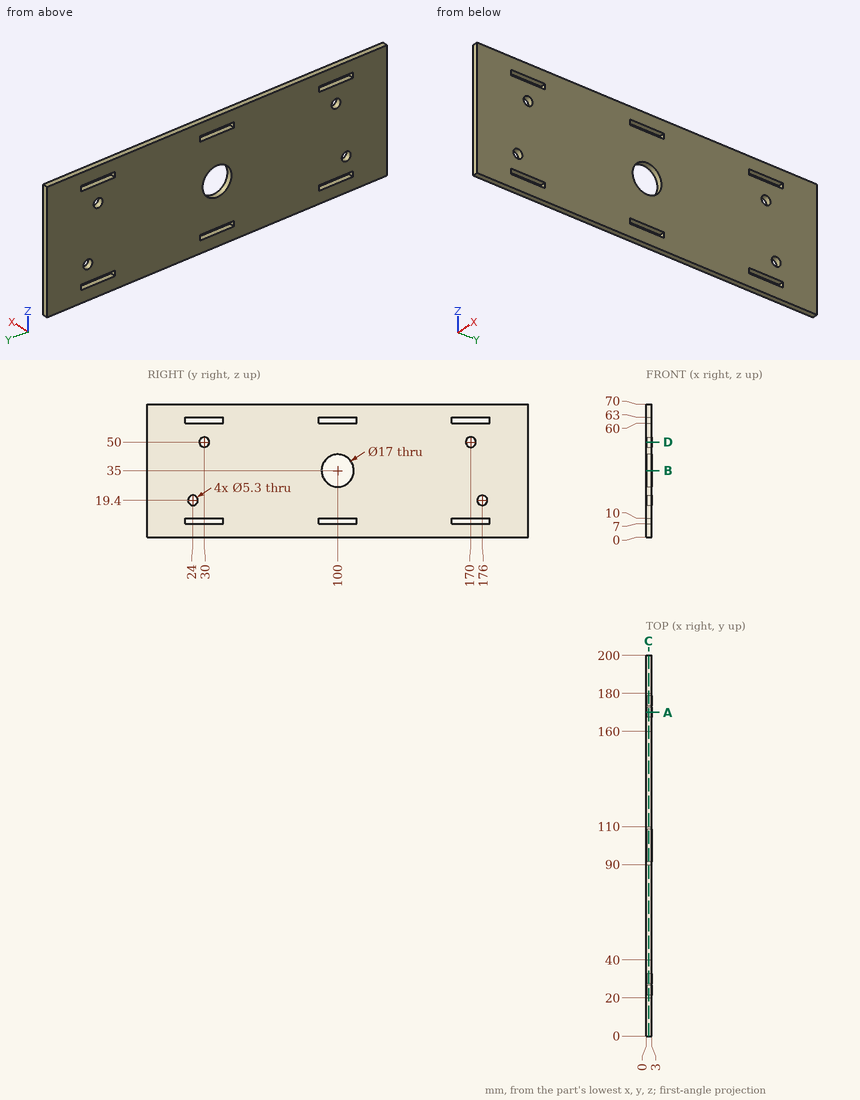
Could you check a few things on this drawing? It's one solid part, dimensions in mm from its lowest x, y, z. Coordinates: 2 decimals unless noted, no trailing zeros. Loops run counter-clockwise (first coordinate to the right, second up) from the corner with the lowest first, then second, coordinate; pieces in that order, holes last.
1. Imagine slicing it at B-B (z = 35). Please give me the cut outline in (x, y), and give its area (3 significant figures).
2. Imagine slicing it at A-A (y = 170). Please give me the cut outline in (x, z), and give its area (3 significant figures).
3. I need wall thicknesses on L1, parallel to Z at x = 1.85, y = 38.5; L2, parallel to Y at x = 1.3, z = 19.4; L3, parallel to Y at x = 1.85, z = 61. Which ranges of each line are inside material? Lowest first, please.
4. Imagine slicing it at D-D (z = 50). Please give me the cut outline in (x, y).
5. Imagine slicing it at C-C (x = 1.35). Give the number of separate pieces and of enclosed holes in the cut face, and give its area (3 significant figures).
Computed values:
1. outline: (0, 0) - (3, 0) - (3, 91.5) - (0, 91.5) - close; (0, 108.5) - (3, 108.5) - (3, 200) - (0, 200) - close
1. area: 549 mm2
2. outline: (0, 0) - (3, 0) - (3, 7) - (0, 7) - close; (0, 10) - (3, 10) - (3, 47.35) - (0, 47.35) - close; (0, 52.65) - (3, 52.65) - (3, 60) - (0, 60) - close; (0, 63) - (3, 63) - (3, 70) - (0, 70) - close
2. area: 176 mm2
3. L1: z = 0 to 7, 10 to 60, 63 to 70
3. L2: y = 0 to 21.35, 26.65 to 173.35, 178.65 to 200
3. L3: y = 0 to 20, 40 to 90, 110 to 160, 180 to 200
4. outline: (0, 0) - (3, 0) - (3, 27.35) - (0, 27.35) - close; (0, 32.65) - (3, 32.65) - (3, 167.35) - (0, 167.35) - close; (0, 172.65) - (3, 172.65) - (3, 200) - (0, 200) - close
5. separate pieces: 1
5. enclosed holes: 11
5. area: 13,300 mm2
